The listing builds one solid part. Answer for the finished solid, in the listing's coordinates (mm). Coordinates: 2 decimals unless noted, no trailing zeros. Write each loop counter-clockwise with the first axis right and the second up, starting at its lowest first coordinate (ties: lowest second). Pieces come first, ordered by that corner, then holes.
(1) The part is cut by section A-A on y = 3.65. Determine the outline of the cut face in (x, z).
(2) Straight lines are drawn through the part: line 1 (X direction, y = 0.95, z = -2); line 2 (Z direction, x = 63, y = 4.1); line 3 (Z direction, x = 72, y = 4.05). For each, find the intervals that lie inside material, in ascending order.
(3) Given P1, Ø3, axis at x = 86, y = 3, coming from the -Z side; P2, Ø1.5, axis at x = -103, y = 3.5, coming from the -Z side, each flat-ended and moving along its own axis, determine where each tip first touches the part or whether it passes through.
Autodesk Inventor part; units mm, degrees
ref_plane "YZ Plane" through (0, 0, 0) normal (1, 0, 0) x (0, 1, 0)
ref_plane "XZ Plane" through (0, 0, 0) normal (0, 1, 0) x (-1, 0, 0)
ref_plane "XY Plane" through (0, 0, 0) normal (0, 0, 1) x (1, 0, 0)
sketch "スケッチ1" plane through (0, 0, 0) normal (0, 1, 0) x (-1, 0, 0)
  line L0 (150, -25) -> (-150, -25)
  line L1 (-150, -25) -> (-150, 25)
  line L2 (-150, 25) -> (150, 25)
  line L3 (150, 25) -> (150, -25)
  line L4 (150, -25) -> (-150, 25) construction
  line L5 (-150, -25) -> (150, 25) construction
  line L6 (150, -25) -> (70, -25)
  line L7 (70, -25) -> (70, -60)
  line L8 (70, -60) -> (150, -60)
  line L9 (150, -60) -> (150, -25)
  line L10 (0, 25) -> (0, -116.583)
  line L11 (-70, -25) -> (-70, -60)
  line L12 (-70, -60) -> (-150, -60)
  line L13 (-150, -60) -> (-150, -25)
  point P0 (0, 0)
  dimension "d0" = 300
  dimension "d1" = 50
  dimension "d7" = 80
  dimension "d8" = 35
extrude "押し出し1" add sketch "スケッチ1" along normal blind 5 contours L0 L10 L2 L3 | L0 L1 L2 L10
chamfer "面取り1" distance 5 angle 45 1 edges at (0, 5, -25)
sketch "スケッチ4" plane through (0, 5, 0) normal (0, 1, 0) x (1, 0, 0)
  line L0 (48, 20) -> (40, 20)
  line L1 (40, 20) -> (40, -5)
  line L2 (40, -5) -> (48, -5)
  line L3 (48, -5) -> (48, 20)
  line L4 (43.5, 0) -> (44.5, 0)
  line L5 (44.5, 0) -> (44.5, 15)
  line L6 (44.5, 15) -> (43.5, 15)
  line L7 (43.5, 15) -> (43.5, 0)
  line L8 (-150, 20) -> (150, 20)
  point P0 (0, 0)
  point P1 (44, 0)
  point P2 (44, -5)
  point P3 (43.5, 7.5)
  point P4 (40, 7.5)
  dimension "d12" = 8
  dimension "d13" = 25
  dimension "d14" = 1
  dimension "d15" = 15
  dimension "d22" = 40
extrude "押し出し4" cut sketch "スケッチ4" against normal through all contours L7 L6 L5 L4
properties part number "HoriMove" material "スタイロフォームIB"
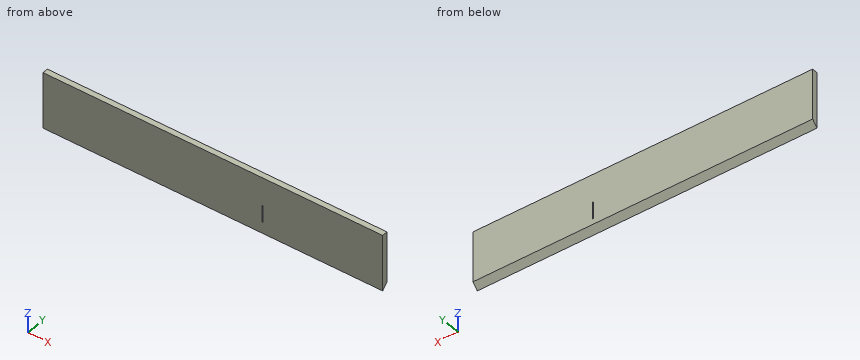
Model answer:
1. outline: (-150, -21.35) - (150, -21.35) - (150, 25) - (-150, 25) - close; hole (43.5, -15) - (44.5, -15) - (44.5, 0) - (43.5, 0) - close
2. line 1: x = -150 to 43.5, 44.5 to 150
2. line 2: z = -20.9 to 25
2. line 3: z = -20.95 to 25
3. P1: stops at z = -23.5
3. P2: stops at z = -22.25
